The listing builds one solid part. Answer for the finished solid, in the listing's coordinates (mm). A direction names the side the tool comes from. Coordinates: 2 decimals unless noted, no trailing zeros. Order: outer loops, then holes, each group sorted by start corner. A loop starts at its lowest first (then second) coordinate and runs counter-clockwise, first axis right, second up. Notation, with made-up numbers: (-39.5, 48) - (-31.5, 48) arc R32 cw to (-31.5, 77) - close; hole circle Ø5 at (85.5, 72). An arc over 180 degrees is marked (long way). Use one line per item in the form item = value. Start each with the question number.
Item 1: Section D-D, the plane x = -5.5 is taken. Write down the section's boundary in (y, z), and give its area (3 significant figures).
Item 2: Section C-C, the plane z = -16 is taken. Write down the section's boundary in (x, y).
Item 3: Section A-A, the plane y = 0 is taken. Write down the section's boundary in (x, z).
Item 4: Consider line 1 along Z through (x, y) = (-8, -11.5); line 2 along Z through (x, y) = (-6, 6.5); line 3 along Y through (x, z) = (-1.5, -3). Determine where each line is inside the solid, lowest interval first. Write a range as [from, to].
Item 5: A tool of negligible diameter and unlimited length cuts with its end or side. For faces 1 (the cylindrical face through (-0.54, -2.44, -13.34)), 2 (the flat face through (0, -21, 20)), from which of +Z, -Z, +X, -X, +Y, -Y can it reach the whole face along a straight path? Write none if from no direction.
from build123d import *

# Parameters (mm, degrees)
SKETCH_1_W      = 42
SKETCH_1_H      = 42
SKETCH_1_R      = 11.5
SKETCH_1_R_2    = 2.5
EXTRUDE_1_DEPTH = 40
SKETCH_1_3_R    = 11.5
SKETCH_1_3_R_2  = 2.5
EXTRUDE_2_DEPTH = 2
SKETCH_1_4_R    = 2.5
EXTRUDE_3_DEPTH = 25


with BuildPart() as part:
    # Sketch 1 → Extrude 1 (new body)
    # profile 1 of 3: a face of its own
    with BuildSketch(Plane.XY):
        Rectangle(SKETCH_1_W, SKETCH_1_H)
        Circle(SKETCH_1_R, mode=Mode.SUBTRACT)
    # profile 2 of 3: a face of its own
    with BuildSketch(Plane.XY):
        Circle(SKETCH_1_R)
        Circle(SKETCH_1_R_2, mode=Mode.SUBTRACT)
    # profile 3 of 3: a face of its own
    with BuildSketch(Plane.XY):
        Circle(SKETCH_1_R_2)
    extrude(amount=EXTRUDE_1_DEPTH)

    # Sketch 1_3 → Extrude 2 (add)
    # profile 1 of 2: a face of its own
    with BuildSketch(Plane.XY):
        Circle(SKETCH_1_3_R)
        Circle(SKETCH_1_3_R_2, mode=Mode.SUBTRACT)
    # profile 2 of 2: a face of its own
    with BuildSketch(Plane.XY):
        Circle(SKETCH_1_3_R_2)
    extrude(amount=-EXTRUDE_2_DEPTH)

    # Sketch 1_4 → Extrude 3 (add)
    with BuildSketch(Plane.XY):
        Circle(SKETCH_1_4_R)
    extrude(amount=-EXTRUDE_3_DEPTH)


solid = part.part
Response:
q1.outline = (-21, 0) - (-10.1, 0) - (-10.1, -2) - (10.1, -2) - (10.1, 0) - (21, 0) - (21, 40) - (-21, 40) - close
q1.area = 1,720 mm2
q2.outline = circle Ø5 at (0, 0)
q3.outline = (-21, 0) - (-11.5, 0) - (-11.5, -2) - (-2.5, -2) - (-2.5, -25) - (2.5, -25) - (2.5, -2) - (11.5, -2) - (11.5, 0) - (21, 0) - (21, 40) - (-21, 40) - close
q4.line_1 = [0, 40]
q4.line_2 = [-2, 40]
q4.line_3 = [-2, 2]
q5.face_1 = -Z
q5.face_2 = +Z, -Z, +X, -X, -Y
